from build123d import *

# Parameters (mm, degrees)
F0_W     = 5
F0_H     = 20
F0_W_2   = 20
F1_DEPTH = 20
F3_START = -5
F3_DEPTH = 20


with BuildPart() as f1:
    # F0 (on Top) → F1 (new body)
    with BuildSketch(Plane.XY):
        with Locations((2.5, 10)):
            Rectangle(F0_W, F0_H)
        with Locations((27.5, 10)):
            Rectangle(F0_W, F0_H)
        with Locations((15, 10)):
            Rectangle(F0_W_2, F0_H)
    extrude(amount=F1_DEPTH)

    # F2 (on face) → F3 (cut)
    with BuildSketch(Plane.YZ.offset(30).offset(F3_START)):
        Polygon((0, 5), (15, 20), (0, 20), align=None)
    extrude(amount=-F3_DEPTH, mode=Mode.SUBTRACT)


solid = f1.part
Part model, mm, in its own coordinate system. A direction names the side the tool comes from. Coordinates: 2 decimals unless noted, no trailing zeros. Write each loop counter-clockwise with the first axis right and the second up, starting at its lowest first coordinate (ties: lowest second). Pieces come first, ordered by that corner, then holes. Notation, with made-up numbers: M 70.25,65 L 88.25,65 A15 cw 88.25,87 Z; hole C 16,40 d8. An arc over 180 degrees is marked long. Return JSON: item names as keys, results as strings.
1. 3-axis set-ups, long thin cutter, end or side, ignore diameter. For faces 5 (the face through (5, 6, 14)), 6 (the face through (11, 0, 3)): which of +Z, -Z, +X, -X, +Y, -Y reach the whole face in a straight line?
Determined:
{"face 5": "+Z, -Y", "face 6": "+Z, -Z, +X, -X, -Y"}
2. Saw through at B-B, the plane z = 17.5. Write the cut outline in (x, y).
Determined:
{"outline": "M 0,0 L 5,0 L 5,12.5 L 25,12.5 L 25,0 L 30,0 L 30,20 L 0,20 Z"}
3. Saw through at A-A, the plane y = 12.75. Write the cut outline in (x, z).
Determined:
{"outline": "M 0,0 L 30,0 L 30,20 L 25,20 L 25,17.75 L 5,17.75 L 5,20 L 0,20 Z"}
4. Pull direction X, two halves, no side cores. Call faces 1 (the face through (25, 6, 14)), 2 (the face through (30, 10, 10)), 3 (the face through (15, 7, 12)), 4 (the face through (0, 10, 10)): pulls with the +X half, pulls with the -X half, needs draft (parallel to the pull), parting line crosses it, or undercut.
Determined:
{"face 1": "undercut", "face 2": "pulls with the +X half", "face 3": "undercut", "face 4": "pulls with the -X half"}
5. Probe L1, parallel to X at y = 7.5, z = 17.75; L2, parallel to Z at x = 11.5, y = 13.75; L3, parallel to Y at x = 13.75, z = 8.75. List the from-to ranges inside material, lowest first.
Determined:
{"L1": "0 to 5, 25 to 30", "L2": "0 to 18.75", "L3": "3.75 to 20"}
6. Flat gauge pin, fed straight in: pin 1 Ø5 at (x, y) = (15.5, 5.5) entering from +Z. Where does the tip first touch, or does it go through?
Determined:
{"pin 1": "z = 13"}
7. Saw through at C-C, the plane x = 21.75. Write the cut outline in (y, z).
Determined:
{"outline": "M 0,0 L 20,0 L 20,20 L 15,20 L 0,5 Z"}
